For this review, take the finished solid that the model builds, in its own axes (mm). A direction names the side the tool comes from. Give positions to 0.01 mm unless a question says otherwise; leave off trailing zeros. Loops run counter-clockwise (first coordinate to the right, second up) from the corner with the lowest first, then second, coordinate; pieces in that order, holes last. Notation, with made-up numbers: (18, 55) - (31, 55) arc R8 cw to (31, 60) - close; hole circle Ø1 at (32.5, 77.25). An arc over 180 degrees is marked (long way). Answer in a Markdown table with one row per item.
Autodesk Inventor part; units mm, degrees
ref_plane "YZ Plane" through (0, 0, 0) normal (1, 0, 0) x (0, 1, 0)
ref_plane "XZ Plane" through (0, 0, 0) normal (0, 1, 0) x (-1, 0, 0)
ref_plane "XY Plane" through (0, 0, 0) normal (0, 0, 1) x (1, 0, 0)
sketch "Skizze1" plane through (0, 0, 0) normal (0, 0, 1) x (1, 0, 0)
  line L0 (-27.5, -27.5) -> (27.5, -27.5)
  line L1 (27.5, -27.5) -> (27.5, 27.5)
  line L2 (27.5, 27.5) -> (-27.5, 27.5)
  line L3 (-27.5, 27.5) -> (-27.5, -27.5)
  line L4 (-27.5, -27.5) -> (27.5, 27.5) construction
  line L5 (27.5, -27.5) -> (-27.5, 27.5) construction
  point P0 (0, 0)
  dimension "d0" = 55
  dimension "d1" = 55
extrude "Extrusion1" add sketch "Skizze1" against normal blind 12
sketch "Skizze2" plane through (0, 0, -12) normal (0, 0, -1) x (-1, 0, 0)
  line L0 (27.5, 27.5) -> (-27.5, 27.5)
  circle A0 centre (-27.5, 27.5) radius 10
  line L1 (27.5, -27.5) -> (27.5, 27.5)
  circle A1 centre (27.5, 27.5) radius 10
  circle A2 centre (27.5, -27.5) radius 10
  circle A3 centre (-27.5, -27.5) radius 10
  point P0 (0, 0)
  dimension "d4" = 20
extrude "Extrusion2" cut sketch "Skizze2" against normal blind 7
sketch "Skizze3" plane through (0, 0, -12) normal (0, 0, -1) x (-1, 0, 0)
  arc A0 (27.5, -17.5) -> (17.5, -27.5) centre (27.5, -27.5) ccw
  line L0 (27.5, -17.5) -> (27.5, 17.5)
  arc A1 (17.5, 27.5) -> (27.5, 17.5) centre (27.5, 27.5) ccw
  line L1 (17.5, 27.5) -> (-17.5, 27.5)
  arc A2 (-27.5, 17.5) -> (-17.5, 27.5) centre (-27.5, 27.5) ccw
  line L2 (-27.5, 17.5) -> (-27.5, -17.5)
  arc A3 (-17.5, -27.5) -> (-27.5, -17.5) centre (-27.5, -27.5) ccw
  line L3 (-17.5, -27.5) -> (17.5, -27.5)
  line L4 (-17.0119, 27) -> (17.0119, 27)
  arc A4 (17.0119, 27) -> (27, 17.0119) centre (27.5, 27.5) ccw
  line L5 (27, 17.0119) -> (27, -17.0119)
  arc A5 (27, -17.0119) -> (17.0119, -27) centre (27.5, -27.5) ccw
  line L6 (17.0119, -27) -> (-17.0119, -27)
  arc A6 (-17.0119, -27) -> (-27, -17.0119) centre (-27.5, -27.5) ccw
  line L7 (-27, -17.0119) -> (-27, 17.0119)
  arc A7 (-27, 17.0119) -> (-17.0119, 27) centre (-27.5, 27.5) ccw
  point P0 (0, 0)
  dimension "d7" = 0.5
extrude "Extrusion3" add sketch "Skizze3" along normal blind 31 contours L4 A4 L5 A5 L6 A6 L7 A7
sketch "Skizze4" plane through (0, 0, -43) normal (0, 0, -1) x (-1, 0, 0)
  arc A0 (17.0119, 27) -> (27, 17.0119) centre (27.5, 27.5) ccw
  line L0 (27, 17.0119) -> (27, -17.0119)
  arc A1 (27, -17.0119) -> (17.0119, -27) centre (27.5, -27.5) ccw
  line L1 (17.0119, -27) -> (-17.0119, -27)
  arc A2 (-17.0119, -27) -> (-27, -17.0119) centre (-27.5, -27.5) ccw
  line L2 (-27, -17.0119) -> (-27, 17.0119)
  arc A3 (-27, 17.0119) -> (-17.0119, 27) centre (-27.5, 27.5) ccw
  line L3 (-17.0119, 27) -> (17.0119, 27)
  arc A4 (27.5, -17.5) -> (17.5, -27.5) centre (27.5, -27.5) ccw
  line L4 (27.5, -17.5) -> (27.5, 17.5)
  arc A5 (17.5, 27.5) -> (27.5, 17.5) centre (27.5, 27.5) ccw
  line L5 (17.5, 27.5) -> (-17.5, 27.5)
  arc A6 (-27.5, 17.5) -> (-17.5, 27.5) centre (-27.5, 27.5) ccw
  line L6 (-27.5, 17.5) -> (-27.5, -17.5)
  arc A7 (-17.5, -27.5) -> (-27.5, -17.5) centre (-27.5, -27.5) ccw
  line L7 (-17.5, -27.5) -> (17.5, -27.5)
  point P0 (0, 0)
extrude "Extrusion4" add sketch "Skizze4" along normal blind 10 contours A0 L0 A1 L1 A2 L2 A3 L3 | A4 L7 A7 L6 A6 L5 A5 L4
sketch "Skizze6" plane through (0, 0, 0) normal (0, 0, 1) x (1, 0, 0)
  line L0 (-23.55, -23.55) -> (23.55, -23.55)
  line L1 (23.55, -23.55) -> (23.55, 23.55)
  line L2 (23.55, 23.55) -> (-23.55, 23.55)
  line L3 (-23.55, 23.55) -> (-23.55, -23.55)
  line L4 (-23.55, -23.55) -> (23.55, 23.55) construction
  line L5 (23.55, -23.55) -> (-23.55, 23.55) construction
  circle A0 centre (-23.55, 23.55) radius 2
  circle A1 centre (23.55, 23.55) radius 2
  circle A2 centre (23.55, -23.55) radius 2
  circle A3 centre (-23.55, -23.55) radius 2
  point P0 (0, 0)
  dimension "d12" = 4
  dimension "d13" = 47.1
  dimension "d14" = 47.1
extrude "Extrusion5" cut sketch "Skizze6" along normal through all both and the other way through all contours L3 A3 L0 | L0 A3 L3 | A2 L1 L0 | L0 L1 A2 | A0 L2 L3 | L3 L2 A0 | A1 L2 L1 | L1 L2 A1
fillet "Rundung1" radius 2 4 edges at (27.5, 27.5, -2.5) (-27.5, 27.5, -2.5) (27.5, -27.5, -2.5) (-27.5, -27.5, -2.5)
sketch "Skizze7" plane through (0, 0, 0) normal (0, 0, 1) x (1, 0, 0)
  circle A0 centre (0, 0) radius 19.05
  dimension "d18" = 38.1
extrude "Extrusion6" add sketch "Skizze7" along normal blind 1.6
sketch "Skizze8" plane through (0, 0, 1.6) normal (0, 0, 1) x (1, 0, 0)
  circle A0 centre (0, 0) radius 3.175
  dimension "d21" = 6.35
extrude "Extrusion7" add sketch "Skizze8" along normal blind 20
sketch "Skizze9" plane through (0, 0, 21.6) normal (0, 0, 1) x (1, 0, 0)
  line L0 (-1.7861, 2.625) -> (1.7861, 2.625)
  line L1 (1.7861, 2.625) -> (1.7861, 3.175)
  line L2 (1.7861, 3.175) -> (-1.7861, 3.175)
  line L3 (-1.7861, 3.175) -> (-1.7861, 2.625)
  circle A0 centre (0, 0) radius 3.175
  point P0 (0, 3.175)
  dimension "d29" = 5.8
extrude "Extrusion8" cut sketch "Skizze9" against normal blind 15 contours A0 L0 | L3 L2 A0 | A0 L2 L1 picked at (-0.4105, 2.7255)
properties part number "MC18_Motor"
1. Mouldability with a two-part tool opening along Y and no side actions: class faces 5 (the face through (22.076, 24.902, -2.465)), 6 (the face through (20.35, -20.51, -8.55)), 7 (the face through (-0.41, -3.15, 11.46)), 8 (the face through (-20.15, 20, -27.28)) as released by +Y, released by -Y, zero draft, split by the parting line, or undercut.
Values:
| item | result |
|---|---|
| face 5 | undercut |
| face 6 | released by -Y |
| face 7 | split by the parting line |
| face 8 | released by +Y |
2. We need section C-C, the plane x = 0. Give the boundary of the cut face in (y, z) (3 decimals).
Values:
| item | result |
|---|---|
| outline | (-27.5, -53) - (27.5, -53) - (27.5, -43) - (27, -43) - (27, -12) - (27.5, -12) - (27.5, 0) - (19.05, 0) - (19.05, 1.6) - (3.175, 1.6) - (3.175, 6.6) - (2.625, 6.6) - (2.625, 21.6) - (-3.175, 21.6) - (-3.175, 1.6) - (-19.05, 1.6) - (-19.05, 0) - (-27.5, 0) - (-27.5, -12) - (-27, -12) - (-27, -43) - (-27.5, -43) - close |
3. We need section D-D, the plane y = 11.5. Give the boundary of the cut face in (x, z), and give its area (3 significant figures).
Values:
| item | result |
|---|---|
| outline | (-27.5, -53) - (27.5, -53) - (27.5, -43) - (27, -43) - (27, -12) - (27.5, -12) - (27.5, 0) - (15.19, 0) - (15.19, 1.6) - (-15.19, 1.6) - (-15.19, 0) - (-27.5, 0) - (-27.5, -12) - (-27, -12) - (-27, -43) - (-27.5, -43) - close |
| area | 2,930 mm^2 |
4. For faces 1 (the face through (-20, -20.15, -27.28)), 2 (the face through (0, 2.625, 14)), 3 (the face through (-20.35, 20.51, -8.55)), 4 (the face through (-19, 6, 0)), list the 3-axis set-ups (+Z, -Z, +X, -X, +Y, -Y) from which the entire face can be reached by the end or side of a thin tool; tool diameter is ignored.
Values:
| item | result |
|---|---|
| face 1 | -X, -Y |
| face 2 | +Z, +X, -X, +Y |
| face 3 | -Z, -X, +Y |
| face 4 | +Z |
5. Clearance check with flat-ended pins moving along their axes: pin 1 (6 mm diameter, centred on x = 16.5, z = -25.5, fed in from -Y); pin 2 (9.5 mm diameter, centred on y = 6, z = -23, fed in from -X); pin 3 (4 mm diameter, centred on x = -0.5, z = 17.5, fed in from +Y) (3 decimals); pin 4 (3.5 mm diameter, centred on x = 23.55, y = -23.55, fed in from -Z). State where each tip first meets the part, or that it passes through.
Values:
| item | result |
|---|---|
| pin 1 | stops at y = -27 |
| pin 2 | stops at x = -27 |
| pin 3 | stops at y = 2.625 |
| pin 4 | passes through |
6. We need section A-A, the plane y = -23.55. Give the boundary of the cut face in (x, z), and give its area (3 significant figures).
Values:
| item | result |
|---|---|
| outline | (-27.5, -5) - (-25.55, -5) - (-25.55, 0) - (-27.5, 0) - close; (-21.55, -5) - (-18.31, -5) - (-18.31, -12) - (-17.77, -12) - (-17.77, -43) - (-18.31, -43) - (-18.31, -53) - (18.31, -53) - (18.31, -43) - (17.77, -43) - (17.77, -12) - (18.31, -12) - (18.31, -5) - (21.55, -5) - (21.55, 0) - (-21.55, 0) - close; (25.55, -5) - (27.5, -5) - (27.5, 0) - (25.55, 0) - close |
| area | 1,960 mm^2 |
7. Wall thickness on line 1 (Y direction, x = -23.55, z = -1.1); line 2 (Z direction, x = 16, y = -11); line 3 (Z direction, x = -9.5, y = -6.5): over which ranges is each line inside the solid? List them lowest first. Write a range as [from, to].
Values:
| item | result |
|---|---|
| line 1 | y = [-27.5, -25.55], [-21.55, 21.55], [25.55, 27.5] |
| line 2 | z = [-53, 0] |
| line 3 | z = [-53, 1.6] |
8. We need section B-B, the plane z = -26. Give the boundary of the cut face in (x, y), and give its area (3 significant figures).
Values:
| item | result |
|---|---|
| outline | (-27, -17.01) arc R10.5 cw to (-17.01, -27) - (17.01, -27) arc R10.5 cw to (27, -17.01) - (27, 17.01) arc R10.5 cw to (17.01, 27) - (-17.01, 27) arc R10.5 cw to (-27, 17.01) - close |
| area | 2,610 mm^2 |
